The drawing under review shows one solid part. Ordinate dimensions are in mm from its lowest x, y, z. Round coordinates to 2 decimals unless told otherwise and drop trailing zeros. Order: outer loops, then holes, each group sorted by start corner. A loop starts at its lowest first (then second) coordinate and runs counter-clockwise, first axis right, second up.
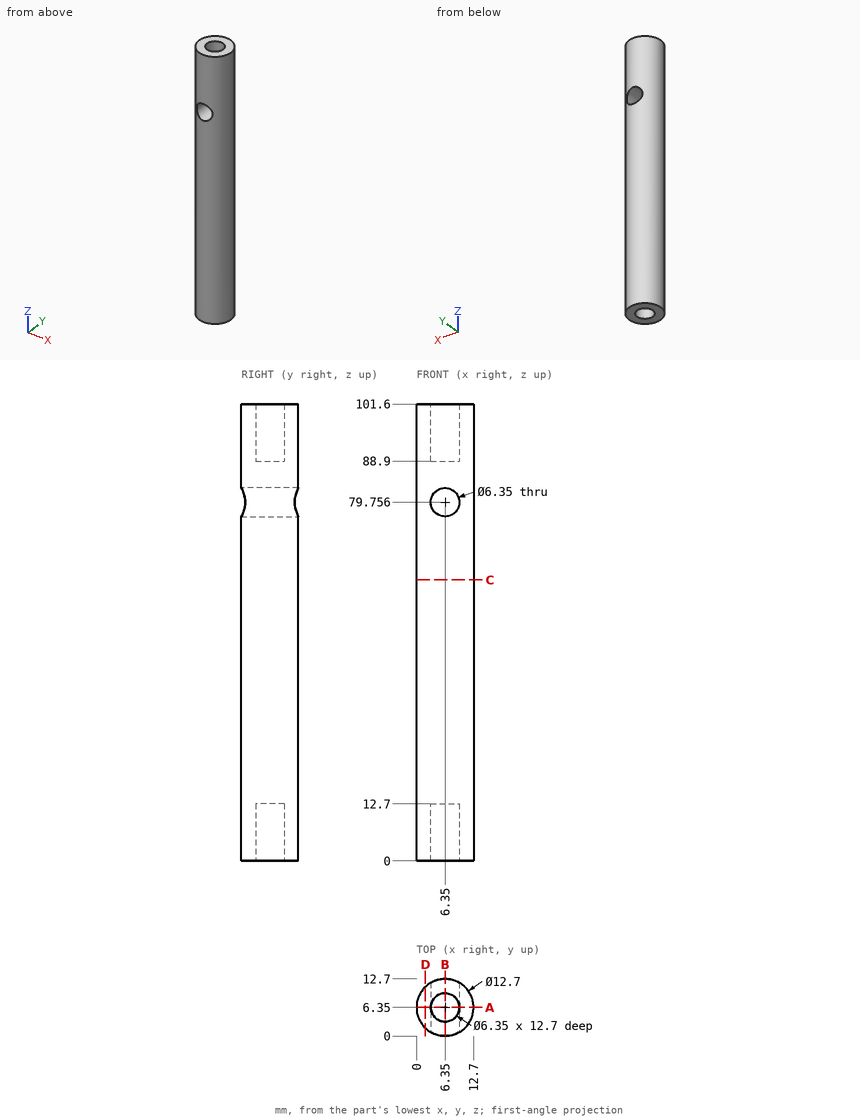
Q1. Wall thickness on line 1 (Y direction, x = 6.5, z = 4.5); line 2 (Z direction, x = 6.25, y = 9.25); line 3 (Y direction, x = 8.5, z = 11.5): over which ranges is each line inside the solid? List them lowest first.
Q2. Take a section at B-B, the plane x = 6.35. State the section outline as (y, z) points (3 decimals).
Q3. Clearance check with flat-ended pins moving along their axes: pin 1 (2 mm diameter, centred on x = 8.5, y = 5, fed in from -Z); pin 2 (3 mm diameter, centred on y = 9.5, z = 74, fed in from +X); pin 3 (5 mm diameter, centred on x = 10.5, z = 40.5, fed in from -Y); pin 4 (1 mm diameter, centred on x = 8.5, y = 5, fed in from -Z). State where each tip first meets the part, or that it passes through.
Q4. Take a section at D-D, the plane x = 2. State the section outline as (y, z) points.
Q5. Take a section at A-A, the plane y = 6.35. State the section outline as (x, z) points (3 decimals).
Q6. Take a section at C-C, the plane z = 62.5. State the section outline as (x, y) points.
Working result:
1. line 1: y = 0 to 3.18, 9.52 to 12.7
1. line 2: z = 12.7 to 76.58, 82.93 to 88.9
1. line 3: y = 0.38 to 4.01, 8.69 to 12.32
2. outline: (0, 0) - (3.175, 0) - (3.175, 12.7) - (9.525, 12.7) - (9.525, 0) - (12.7, 0) - (12.7, 76.581) - (0, 76.581) - close; (0, 82.931) - (12.7, 82.931) - (12.7, 101.6) - (9.525, 101.6) - (9.525, 88.9) - (3.175, 88.9) - (3.175, 101.6) - (0, 101.6) - close
3. pin 1: stops at z = 0
3. pin 2: stops at x = 12.48
3. pin 3: stops at y = 0.22
3. pin 4: stops at z = 12.7
4. outline: (1.72, 0) - (10.98, 0) - (10.98, 101.6) - (1.72, 101.6) - close
5. outline: (0, 0) - (3.175, 0) - (3.175, 12.7) - (9.525, 12.7) - (9.525, 0) - (12.7, 0) - (12.7, 101.6) - (9.525, 101.6) - (9.525, 88.9) - (3.175, 88.9) - (3.175, 101.6) - (0, 101.6) - close; hole circle Ø6.35 at (6.35, 79.756)
6. outline: circle Ø12.7 at (6.35, 6.35)
